The model under review builds one solid part; all positions refer to its coordinate system, in mm. A direction names the side the tool comes from. Coordinates: 2 decimals unless noted, no trailing zeros. Loops run counter-clockwise (first coordinate to the right, second up) from the corner with the lowest first, then second, coordinate; pieces in that order, holes last. Notation, with made-up numbers: (-10, 3) - (2, 3) arc R23 cw to (2, 25) - close; hole circle Ø10 at (48, 85). An arc over 180 degrees is marked (long way). Use a Markdown table: item, result. Add a question column.
1) Add section B-B, the plane z = 9. Give the boundary of the cut face in (x, y).
2) The part is to be moulded in two halves that separate along X. For faces 1 (the cylindrical face through (23.846, 0.493, 7.509)), 2 (the cylindrical face through (-19, 8, 0)), 3 (the flat face through (0, 2, 0)), say which applies: pulls with the +X half, pulls with the -X half, needs draft (parallel to the pull), parting line crosses it, or undercut.
3) To check wall thickness, follow L1, parallel to Z at x = 0, y = 4.25; L2, parallel to Y at x = -4, z = -5; L3, parallel to Z at x = -11.5, y = 4.5. State the ranges of each line that lie inside material, in increasing order. Write a range as [from, to].
4) Add section D-D, the plane x = 13. Give the boundary of the cut face in (y, z).
5) Add section A-A, the plane y = 9.5. Give the boundary of the cut face in (x, z), and give its area (3 significant figures).
6) For faces 4 (the flat face through (0, 0, 0)), 5 (the flat face through (-7, 1, 0)), 6 (the flat face through (1, 2.8, 0.1)), list the 3-axis set-ups (+Z, -Z, +X, -X, +Y, -Y) from which the entire face can be reached by the end or side of a thin tool; tool diameter is ignored.
7) Add section C-C, the plane x = -4. Give the boundary of the cut face in (y, z).
8) Clearance check with flat-ended pins moving along their axes: pin 1 (3 mm diameter, centred on x = -14.5, y = 11.5, fed in from -Z); pin 2 (1 mm diameter, centred on x = -6.5, z = 10.5, fed in from +Y); pin 3 (14.5 mm diameter, centred on x = -5, z = 8.5, fed in from +Y). State where each tip first meets the part, or that it passes through.
Autodesk Inventor part; units mm, degrees
ref_plane "YZ Plane" through (0, 0, 0) normal (1, 0, 0) x (0, 1, 0)
ref_plane "XZ Plane" through (0, 0, 0) normal (0, 1, 0) x (-1, 0, 0)
ref_plane "XY Plane" through (0, 0, 0) normal (0, 0, 1) x (1, 0, 0)
sketch "スケッチ1" plane through (0, 0, 0) normal (0, 1, 0) x (-1, 0, 0)
  arc A0 (0, -19) -> (0, 19) centre (0, 0) ccw
  line L0 (0, 19) -> (-1, 19)
  line L1 (-1, 19) -> (-1, -19)
  line L2 (-1, -19) -> (0, -19)
  dimension "d0" = 19
  dimension "d1" = 1
  dimension "d2" = 38
extrude "押し出し1" add sketch "スケッチ1" along normal blind 15
sketch "スケッチ2" plane through (0, 15, 0) normal (0, 1, 0) x (1, 0, 0)
  arc A0 (0, 18) -> (0, -18) centre (0, 0) ccw
  line L0 (0, -18) -> (0, 18)
  dimension "d5" = 18
extrude "押し出し2" cut sketch "スケッチ2" against normal blind 14
sketch "スケッチ3" plane through (0, 15, 0) normal (0, 1, 0) x (1, 0, 0)
  line L0 (0, 18) -> (0, -18)
  line L1 (0, -18) -> (2.1384, -18)
  line L2 (2.1384, -18) -> (2.1384, 18)
  line L3 (2.1384, 18) -> (0, 18)
  line L4 (0, 18) -> (0, -18)
  point P0 (0, 0)
  dimension "d13" = 36
extrude "押し出し3" cut sketch "スケッチ3" against normal blind 12
sketch "スケッチ4" plane through (0, 0, 0) normal (0, -1, 0) x (1, 0, 0)
  circle A0 centre (0, 0) radius 25
  dimension "d10" = 50
extrude "押し出し4" add sketch "スケッチ4" against normal blind 1
properties part number "Shield_WeldSupport"
From the geometry:
| question | item | result |
|---|---|---|
| 1 | outline | (-23.32, 0) - (23.32, 0) - (23.32, 1) - (1, 1) - (1, 3) - (0, 3) - (0, 1) - (-15.59, 1) - (-15.59, 15) - (-16.73, 15) - (-16.73, 1) - (-23.32, 1) - close |
| 2 | face 1 | parting line crosses it |
| 2 | face 2 | pulls with the -X half |
| 2 | face 3 | undercut |
| 3 | L1 | z = [-19, -18], [18, 19] |
| 3 | L2 | y = [0, 1] |
| 3 | L3 | z = [-15.12, -13.85], [13.85, 15.12] |
| 4 | outline | (0, -21.35) - (1, -21.35) - (1, 21.35) - (0, 21.35) - close |
| 5 | outline | (0, -19) - (1, -19) - (1, -18) - (0, -18) arc R18 cw to (0, 18) - (1, 18) - (1, 19) - (0, 19) arc R19 ccw to start |
| 5 | area | 60.1 mm^2 |
| 6 | face 4 | +Z, -Z, +X, -X, -Y |
| 6 | face 5 | +Y |
| 6 | face 6 | +Z, -Z, +X, +Y |
| 7 | outline | (0, -24.68) - (1, -24.68) - (1, -18.57) - (15, -18.57) - (15, -17.55) - (1, -17.55) - (1, 17.55) - (15, 17.55) - (15, 18.57) - (1, 18.57) - (1, 24.68) - (0, 24.68) - close |
| 8 | pin 1 | stops at z = -13.86 |
| 8 | pin 2 | stops at y = 1 |
| 8 | pin 3 | stops at y = 3 |
